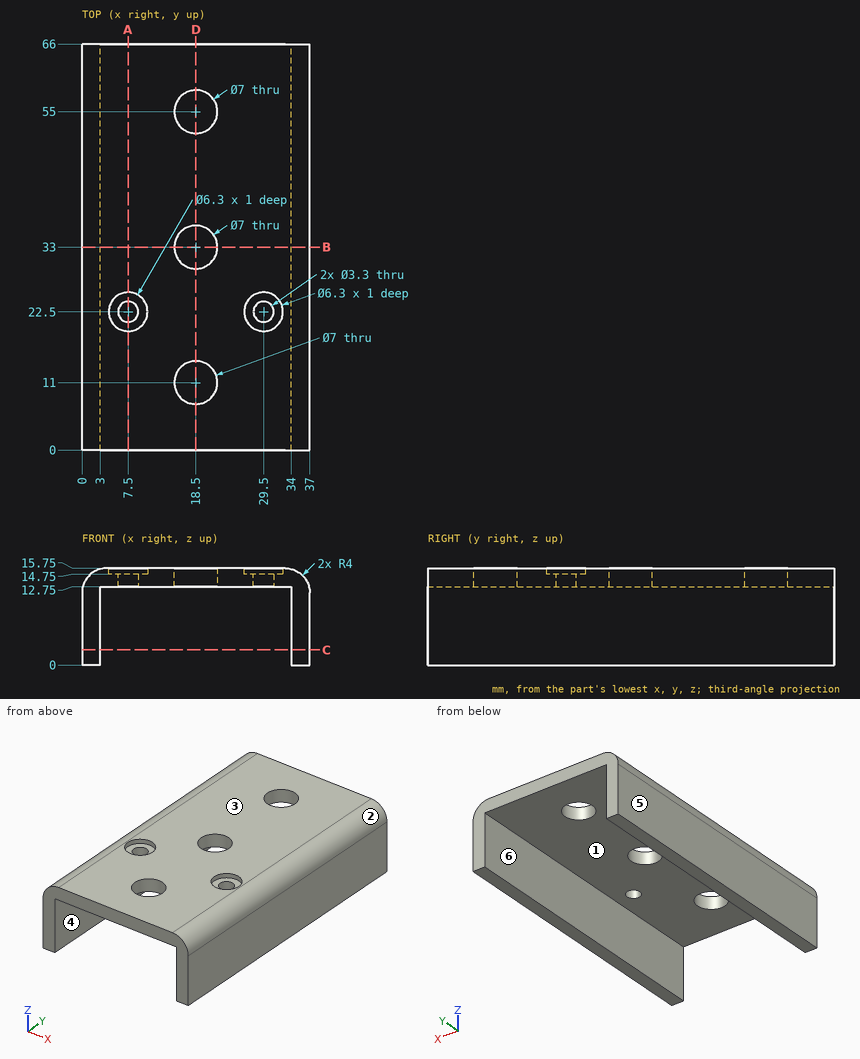
Study the drawing (mm; zero at the part's minimum x, y, z) and answer. A direction names the side the tool comes from. Give positions to 0.01 mm unless a question says otherwise; leave off trailing zeros. Write each loop counter-clockwise with the first axis right and the second up, starting at its lowest first coordinate (ties: lowest second). Pieces come first, ordered by that corner, then holes. Notation, with made-up numbers: (17.5, 68.25) -> (66.5, 68.25) arc R24 ccw to (66.5, 83.25) -> close; hole circle Ø10 at (-6.75, -5.75). An arc over 180 degrees is marked (long way). Answer in a Markdown table with one row per item.
1) Each of these flat-tipped pins is pushed along its axis until it touches: pin 1 Ø4 at (x, y) = (18.5, 11) entering from -Z; pin 2 Ø7 at (x, y) = (29, 23.5) entering from +Z; pin 3 Ø3 at (x, y) = (8, 22.5) entering from +Z; pin 4 Ø3 at (x, y) = (8, 14) entering from -Z. Where does it stop, or does it pass through?
Results list:
| item | result |
|---|---|
| pin 1 | through |
| pin 2 | z = 15.75 |
| pin 3 | z = 14.75 |
| pin 4 | z = 12.75 |
2) Straight lines are drawn through the part: line 1 (Y direction, x = 18.5, z = 13.45); line 2 (X direction, y = 33, z = 6.5); line 3 (Y direction, x = 7.5, z = 13.95). For each, find the intervals that lie inside material, in ascending order. Write a range as [from, to].
Results list:
| item | result |
|---|---|
| line 1 | [0, 7.5], [14.5, 29.5], [36.5, 51.5], [58.5, 66] |
| line 2 | [0, 3], [34, 37] |
| line 3 | [0, 20.85], [24.15, 66] |
3) Determine the mould class of the marked faces 1, 2, 3 and 4 for opening direction X: released by +X, released by -X, zero draft, split by the parting line, or undercut.
Results list:
| item | result |
|---|---|
| face 1 | undercut |
| face 2 | released by +X |
| face 3 | zero draft |
| face 4 | undercut |
4) Section D-D on x = 18.5 is taken. Give the vertices of the cut face in (y, z), plus the area to 3 significant figures.
Results list:
| item | result |
|---|---|
| outline | (0, 12.75) -> (7.5, 12.75) -> (7.5, 15.75) -> (0, 15.75) -> close; (14.5, 12.75) -> (29.5, 12.75) -> (29.5, 15.75) -> (14.5, 15.75) -> close; (36.5, 12.75) -> (51.5, 12.75) -> (51.5, 15.75) -> (36.5, 15.75) -> close; (58.5, 12.75) -> (66, 12.75) -> (66, 15.75) -> (58.5, 15.75) -> close |
| area | 135 mm^2 |
5) Section B-B on y = 33 is taken. Give the vertices of the cut face in (x, z), plus the area to 3 significant figures.
Results list:
| item | result |
|---|---|
| outline | (0, 0) -> (3, 0) -> (3, 12.75) -> (15, 12.75) -> (15, 15.75) -> (4, 15.75) arc R4 ccw to (0, 11.75) -> close; (22, 12.75) -> (34, 12.75) -> (34, 0) -> (37, 0) -> (37, 11.75) arc R4 ccw to (33, 15.75) -> (22, 15.75) -> close |
| area | 160 mm^2 |
6) A tool of negligible diameter and unlimited length cuts with its end or side. For the marked faces 5 and 6, from which of +Z, -Z, +X, -X, +Y, -Y can it reach the whole face along a straight path? Write none if from no direction.
Results list:
| item | result |
|---|---|
| face 5 | +Z, -Z, -X, +Y, -Y |
| face 6 | -Z, +Y, -Y |
7) Section C-C on z = 2.5 is taken. Give the vertices of the cut face in (x, y), plus the area to 3 significant figures.
Results list:
| item | result |
|---|---|
| outline | (0, 0) -> (3, 0) -> (3, 66) -> (0, 66) -> close; (34, 0) -> (37, 0) -> (37, 66) -> (34, 66) -> close |
| area | 396 mm^2 |
8) Section A-A on x = 7.5 is taken. Give the vertices of the cut face in (y, z).
Results list:
| item | result |
|---|---|
| outline | (0, 12.75) -> (20.85, 12.75) -> (20.85, 14.75) -> (19.35, 14.75) -> (19.35, 15.75) -> (0, 15.75) -> close; (24.15, 12.75) -> (66, 12.75) -> (66, 15.75) -> (25.65, 15.75) -> (25.65, 14.75) -> (24.15, 14.75) -> close |
